Model file for the job. Use its own axes, mm. A direction names the side the tool comes from. Round coordinates to 2 decimals unless told otherwise and drop trailing zeros. Loops run counter-clockwise (first coordinate to the right, second up) from the corner with the lowest first, then second, coordinate; pieces in that order, holes last. Notation, with made-up numbers: (-12, 61.25) -> (3, 61.25) arc R12 cw to (3, 80.25) -> close; hole circle Ø2 at (45.5, 44.25). An arc over 180 degrees is marked (long way). Use a Markdown table: item, result.
from build123d import *

# Parameters (mm, degrees)
SKETCH_W      = 600
SKETCH_H      = 10
SKETCH001_W   = 67
SKETCH001_H   = 2.5
SKETCH002_W   = 20
SKETCH002_H   = 1.5
SKETCH003_W   = 13
SKETCH003_H   = 2.5
SKETCH003_W_2 = 1
SKETCH003_H_2 = 3.01


with BuildPart() as part:
    # Sketch → Revolution (revolve)
    with BuildSketch(Plane.XZ):
        with Locations((300, 5)):
            Rectangle(SKETCH_W, SKETCH_H)
    revolve(axis=Axis((0, 0, 0), (1, 0, 0)))

    # Sketch001 → Groove (revolve, cut)
    with BuildSketch(Plane.XZ):
        with Locations((33.5, 8.75)):
            Rectangle(SKETCH001_W, SKETCH001_H)
    revolve(axis=Axis((0, 0, 0), (1, 0, 0)), mode=Mode.SUBTRACT)

    # Sketch002 → Groove001 (revolve, cut)
    with BuildSketch(Plane.XZ):
        with Locations((10, 6.75)):
            Rectangle(SKETCH002_W, SKETCH002_H)
    revolve(axis=Axis((0, 0, 0), (1, 0, 0)), mode=Mode.SUBTRACT)

    # Sketch003 → Groove002 (revolve, cut)
    with BuildSketch(Plane.XZ):
        with Locations((593.5, 8.75)):
            Rectangle(SKETCH003_W, SKETCH003_H)
        with Locations((596.5, 5.995)):
            Rectangle(SKETCH003_W_2, SKETCH003_H_2)
    revolve(axis=Axis((0, 0, 0), (1, 0, 0)), mode=Mode.SUBTRACT)


solid = part.part
Q1. Band-saw the part on D-D, the plane x = 45.5. Give the cut face in (y, z), plus the area to 3 significant figures.
Results list:
| item | result |
|---|---|
| outline | circle Ø15 at (0, 0) |
| area | 177 mm² |
Q2. Band-saw the part on C-C, the plane x = 498.5. Give the cut face in (y, z).
Results list:
| item | result |
|---|---|
| outline | circle Ø20 at (0, 0) |
Q3. Pull direction X, two halves, no side cores. Call faces 1 (the face through (43.829, -0.33, -7.493)), 2 (the face through (67, -7, -4)), 3 (the face through (597, 5, 0)): released by +X, released by -X, zero draft, split by the parting line, or undercut.
Results list:
| item | result |
|---|---|
| face 1 | zero draft |
| face 2 | released by -X |
| face 3 | undercut |
Q4. Flat gauge pins, fed straight in: pin 1 (6 mm diameter, centred on x = 92.5, y = -4.5, fed in from -Z); pin 2 (2 mm diameter, centred on x = 341.5, y = -6, fed in from +Z); pin 3 (2 mm diameter, centred on x = 485.5, y = 7, fed in from +Z). Where does each tip first touch, or does it go through?
Results list:
| item | result |
|---|---|
| pin 1 | stops at z = -9.89 |
| pin 2 | stops at z = 8.66 |
| pin 3 | stops at z = 8 |
Q5. Band-saw the part on A-A, the plane y = 0. Give the cut face in (x, z), plus the area to 3 significant figures.
Results list:
| item | result |
|---|---|
| outline | (0, -6) -> (20, -6) -> (20, -7.5) -> (67, -7.5) -> (67, -10) -> (587, -10) -> (587, -7.5) -> (596, -7.5) -> (596, -4.49) -> (597, -4.49) -> (597, -7.5) -> (600, -7.5) -> (600, 7.5) -> (597, 7.5) -> (597, 4.49) -> (596, 4.49) -> (596, 7.5) -> (587, 7.5) -> (587, 10) -> (67, 10) -> (67, 7.5) -> (20, 7.5) -> (20, 6) -> (0, 6) -> close |
| area | 11,500 mm² |
Q6. Drill centre lines: L1, parallel to X at y = 2.75, z = -5; L2, parallel to X at y = -5.75, z = -2.5; L3, parallel to Y at x = 556, z = -6.5. Where is each one in solid material? Low to high. Write a range as from..to.
Results list:
| item | result |
|---|---|
| L1 | x = 0..596, 597..600 |
| L2 | x = 20..596, 597..600 |
| L3 | y = -7.6..7.6 |
Q7. Tool access for faces 4 (the face through (10, 0, -6)), 5 (the face through (587, -7, -4)), 6 (the face through (596, 5, 0)), 7 (the face through (0, 0, 0)): list every direction of +Z, -Z, +X, -X, +Y, -Y with a clear straight run to the whole face (end or side of a thin tool).
Results list:
| item | result |
|---|---|
| face 4 | -X |
| face 5 | +X |
| face 6 | none |
| face 7 | +Z, -Z, -X, +Y, -Y |
